The model under review builds one solid part; all positions refer to its coordinate system, in mm. Coordinates: 2 decimals unless noted, no trailing zeros. Loops run counter-clockwise (first coordinate to the right, second up) from the corner with the lowest first, then second, coordinate; pieces in that order, holes last. Notation, with made-up numbers: M 62,-6.75 L 89,-6.75 A15 cw 89,16.25 Z; hole C -16.5,19 d8. An arc over 180 degrees is marked long. Use CSV: the item, a comma, the result in double quotes. Start each with the question number.
1. Clearance check with flat-ended pins moving along their axes: P1, Ø1, axis at x = 55.5, z = 1.5, coming from the -Y side; P2, Ø1, axis at y = 98.5, z = 1.5, coming from the -X side; P3, Ø1, axis at x = 43, z = 1.5, coming from the +Y side; P4, Ø1, axis at y = 168, z = 0.5, coming from the +X side. State where each tip first meets the part, or that it passes through.
2. Add section B-B, the plane z = 0.95. State how many separate pieces and enclosed holes the cut face has, then the cut area to 3 significant figures.
3. Add section A-A, the plane y = 176.5. Write out the cut boundary in (x, z).
4. For L1, parallel to X at y = 82.5, z = 0.65; L2, parallel to Y at x = 0, z = 1.25; L3, parallel to X at y = 110, z = 0.9, list the stretches that pass through material, from the lowest coordinate up.
from build123d import *

# Parameters (mm, degrees)
SKETCH_1_R      = 1.6
SKETCH_1_W      = 11
SKETCH_1_H      = 7
SKETCH_1_R_2    = 1.5
EXTRUDE_1_DEPTH = 2


with BuildPart() as part:
    # 草圖1 → 填料-伸長1 (new body)
    with BuildSketch(Plane.XY):
        Polygon((62.5, 0), (62.5, 66), (47.5, 66), (47.5, 101), (61, 101), (61, 150), (40, 200), (34, 200), (34, 157), (17, 157), (17, 200), (-17, 200), (-17, 157), (-34, 157), (-34, 200), (-40, 200), (-61, 150), (-61, 101), (-47.5, 101), (-47.5, 66), (-62.5, 66), (-62.5, 0), align=None)
        with Locations((-18.5, 3)):
            Circle(SKETCH_1_R, mode=Mode.SUBTRACT)
        with Locations((-18.5, 53)):
            Circle(SKETCH_1_R, mode=Mode.SUBTRACT)
        with Locations((39, 3)):
            Circle(SKETCH_1_R, mode=Mode.SUBTRACT)
        with Locations((39, 53)):
            Circle(SKETCH_1_R, mode=Mode.SUBTRACT)
        with Locations((42.5, 156)):
            Circle(SKETCH_1_R, mode=Mode.SUBTRACT)
        with Locations((0, 197.5)):
            Circle(SKETCH_1_R, mode=Mode.SUBTRACT)
        with Locations((37.09943713, 197.209058014)):
            Circle(SKETCH_1_R, mode=Mode.SUBTRACT)
        with Locations((-57.5, 5)):
            Circle(SKETCH_1_R, mode=Mode.SUBTRACT)
        with Locations((-42.5, 61)):
            Circle(SKETCH_1_R, mode=Mode.SUBTRACT)
        with Locations((-42.5, 82.5)):
            Circle(SKETCH_1_R, mode=Mode.SUBTRACT)
        with Locations((-33.75, 97.5)):
            Rectangle(SKETCH_1_W, SKETCH_1_H, mode=Mode.SUBTRACT)
        with Locations((57.5, 5)):
            Circle(SKETCH_1_R, mode=Mode.SUBTRACT)
        with Locations((42.5, 61)):
            Circle(SKETCH_1_R, mode=Mode.SUBTRACT)
        with Locations((0, 93.5)):
            Circle(SKETCH_1_R, mode=Mode.SUBTRACT)
        with Locations((42.5, 82.5)):
            Circle(SKETCH_1_R, mode=Mode.SUBTRACT)
        with Locations((33.75, 97.5)):
            Rectangle(SKETCH_1_W, SKETCH_1_H, mode=Mode.SUBTRACT)
        with Locations((-56.996650272, 147.008451352)):
            Circle(SKETCH_1_R, mode=Mode.SUBTRACT)
        with Locations((-20, 101)):
            Circle(SKETCH_1_R, mode=Mode.SUBTRACT)
        with Locations((-42.5, 156)):
            Circle(SKETCH_1_R, mode=Mode.SUBTRACT)
        with Locations((-37.09943713, 197.209058014)):
            Circle(SKETCH_1_R, mode=Mode.SUBTRACT)
        with Locations((20, 101)):
            Circle(SKETCH_1_R, mode=Mode.SUBTRACT)
        with Locations((56.996650272, 147.008451352)):
            Circle(SKETCH_1_R_2, mode=Mode.SUBTRACT)
        with Locations((0, 152)):
            Circle(SKETCH_1_R, mode=Mode.SUBTRACT)
        with Locations((0, 165.5)):
            Circle(SKETCH_1_R, mode=Mode.SUBTRACT)
        with Locations((47.996650272, 110)):
            Circle(SKETCH_1_R, mode=Mode.SUBTRACT)
        with Locations((11, 147)):
            Circle(SKETCH_1_R, mode=Mode.SUBTRACT)
        with Locations((11, 110)):
            Circle(SKETCH_1_R, mode=Mode.SUBTRACT)
        with Locations((47.996650272, 147)):
            Circle(SKETCH_1_R, mode=Mode.SUBTRACT)
        with Locations((-11, 110)):
            Circle(SKETCH_1_R, mode=Mode.SUBTRACT)
        with Locations((-48, 147)):
            Circle(SKETCH_1_R, mode=Mode.SUBTRACT)
        with Locations((-48, 110)):
            Circle(SKETCH_1_R, mode=Mode.SUBTRACT)
        with Locations((-11, 147)):
            Circle(SKETCH_1_R, mode=Mode.SUBTRACT)
    extrude(amount=EXTRUDE_1_DEPTH)


solid = part.part
Computed:
1,P1,"stops at y = 0"
1,P2,"stops at x = -47.5"
1,P3,"stops at y = 194.05"
1,P4,"stops at x = 53.65"
2,separate pieces,"1"
2,enclosed holes,"32"
2,area,"20,700 mm^2"
3,outline,"M -49.87,0 L -34,0 L -34,2 L -49.87,2 Z; M -17,0 L 17,0 L 17,2 L -17,2 Z; M 34,0 L 49.87,0 L 49.87,2 L 34,2 Z"
4,L1,"x = -47.5 to -44.1, -40.9 to 40.9, 44.1 to 47.5"
4,L2,"y = 0 to 91.9, 95.1 to 150.4, 153.6 to 163.9, 167.1 to 195.9, 199.1 to 200"
4,L3,"x = -61 to -49.6, -46.4 to -12.6, -9.4 to 9.4, 12.6 to 46.4, 49.6 to 61"
